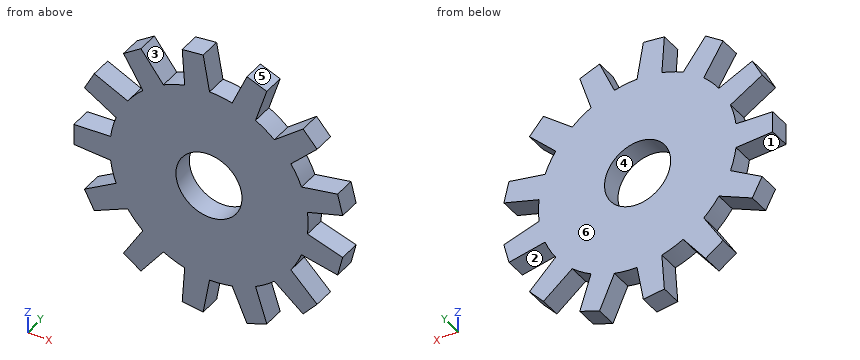
Autodesk Inventor part; units mm, degrees
ref_plane "YZ Plane" through (0, 0, 0) normal (1, 0, 0) x (0, 1, 0)
ref_plane "XZ Plane" through (0, 0, 0) normal (0, 1, 0) x (-1, 0, 0)
ref_plane "XY Plane" through (0, 0, 0) normal (0, 0, 1) x (1, 0, 0)
sketch "Szkic2" plane through (0, 0, 0) normal (0, 1, 0) x (-1, 0, 0)
  circle A0 centre (0, 0) radius 2.5
  circle A1 centre (0, 0) radius 10.25
  line L0 (10.2187, -0.8002) -> (10.2187, 0.8002)
  line L1 (10.2187, -0.8002) -> (7.4401, -0.9459)
  line L2 (10.2187, -0.8002) -> (13.0011, -0.8002) construction
  line L3 (10.2187, 0.8002) -> (7.4401, 0.9459)
  line L4 (10.2187, 0.8002) -> (13.0011, 0.8002) construction
  line L5 (9.4201, 4.0403) -> (7.0275, 2.6201)
  line L6 (8.6763, 5.4575) -> (6.1483, 4.2951)
  line L7 (9.4201, 4.0403) -> (8.6763, 5.4575)
  line L8 (6.4635, 7.9552) -> (5.0049, 5.5858)
  line L9 (5.1463, 8.8644) -> (3.448, 6.6604)
  line L10 (6.4635, 7.9552) -> (5.1463, 8.8644)
  line L11 (2.0261, 10.0477) -> (1.8358, 7.2719)
  line L12 (0.4373, 10.2407) -> (-0.0422, 7.4999)
  line L13 (2.0261, 10.0477) -> (0.4373, 10.2407)
  line L14 (-2.8754, 9.8384) -> (-1.7539, 7.292)
  line L15 (-4.3718, 9.2709) -> (-3.5227, 6.6212)
  line L16 (-2.8754, 9.8384) -> (-4.3718, 9.2709)
  line L17 (-7.1182, 7.3753) -> (-4.9418, 5.6417)
  line L18 (-8.1795, 6.1773) -> (-6.1962, 4.2257)
  line L19 (-7.1182, 7.3753) -> (-8.1795, 6.1773)
  line L20 (-9.7303, 3.2225) -> (-6.9976, 2.6989)
  line L21 (-10.1133, 1.6685) -> (-7.4503, 0.8622)
  line L22 (-9.7303, 3.2225) -> (-10.1133, 1.6685)
  line L23 (-10.1133, -1.6685) -> (-7.4503, -0.8622)
  line L24 (-9.7303, -3.2225) -> (-6.9976, -2.6989)
  line L25 (-10.1133, -1.6685) -> (-9.7303, -3.2225)
  line L26 (-8.1795, -6.1773) -> (-6.1962, -4.2257)
  line L27 (-7.1182, -7.3753) -> (-4.9418, -5.6417)
  line L28 (-8.1795, -6.1773) -> (-7.1182, -7.3753)
  line L29 (-4.3718, -9.2709) -> (-3.5227, -6.6212)
  line L30 (-2.8754, -9.8384) -> (-1.7539, -7.292)
  line L31 (-4.3718, -9.2709) -> (-2.8754, -9.8384)
  line L32 (0.4373, -10.2407) -> (-0.0422, -7.4999)
  line L33 (2.0261, -10.0477) -> (1.8358, -7.2719)
  line L34 (0.4373, -10.2407) -> (2.0261, -10.0477)
  line L35 (5.1463, -8.8644) -> (3.448, -6.6604)
  line L36 (6.4635, -7.9552) -> (5.0049, -5.5858)
  line L37 (5.1463, -8.8644) -> (6.4635, -7.9552)
  line L38 (8.6763, -5.4575) -> (6.1483, -4.2951)
  line L39 (9.4201, -4.0403) -> (7.0275, -2.6201)
  line L40 (8.6763, -5.4575) -> (9.4201, -4.0403)
  arc A2 (7.0275, -2.6201) -> (7.4401, -0.9459) centre (0, 0) ccw
  arc A3 (5.0049, -5.5858) -> (6.1483, -4.2951) centre (0, 0) ccw
  arc A4 (7.4401, 0.9459) -> (7.0275, 2.6201) centre (0, 0) ccw
  arc A5 (6.1483, 4.2951) -> (5.0049, 5.5858) centre (0, 0) ccw
  arc A6 (3.448, 6.6604) -> (1.8358, 7.2719) centre (0, 0) ccw
  arc A7 (-0.0422, 7.4999) -> (-1.7539, 7.292) centre (0, 0) ccw
  arc A8 (-3.5227, 6.6212) -> (-4.9418, 5.6417) centre (0, 0) ccw
  arc A9 (-6.1962, 4.2257) -> (-6.9976, 2.6989) centre (0, 0) ccw
  arc A10 (-7.4503, 0.8622) -> (-7.4503, -0.8622) centre (0, 0) ccw
  arc A11 (-6.9976, -2.6989) -> (-6.1962, -4.2257) centre (0, 0) ccw
  arc A12 (-4.9418, -5.6417) -> (-3.5227, -6.6212) centre (0, 0) ccw
  arc A13 (-1.7539, -7.292) -> (-0.0422, -7.4999) centre (0, 0) ccw
  arc A14 (1.8358, -7.2719) -> (3.448, -6.6604) centre (0, 0) ccw
  dimension "d58" = 5
  dimension "d60" = 20.5
  dimension "d61" = 177
  dimension "d62" = 177
  dimension "d65" = 360
extrude "Wyciągnięcie proste6" add sketch "Szkic2" along normal blind 1.6 contours L0 L1 A2 L39 L40 L38 A3 L36 L37 L35 A14 L33 L34 L32 A13 L30 L31 L29 A12 L27 L28 L26 A11 L24 L25 L23 A10 L21 L22 L20 A9 L18 L19 L17 A8 L15 L16 L14 A7 L12 L13 L11 A6 L9 L10 L8 A5 L6 L7 L5 A4 L3
properties part number "efektor zebatka1"
Geometry: final body of the model. Coordinates: model frame, mm. Face numbers are marked on the shaded views. A direction names the side the tool comes from. Coordinates: 2 decimals unless noted, no trailing zeros. Order: outer loops, then holes, each group sorted by start corner. A loop starts at its lowest first (then second) coordinate and runs counter-clockwise, first axis right, second up. Notation, with made-up numbers: (31, 11.25) -> (43, 11.25) arc R20 ccw to (43, 25.25) -> close; hole circle Ø7 at (62, 89.5). An arc over 180 degrees is marked (long way). Write each question's results on one line, items separated by ' | '. Start each with the question number.
1) Cut plane C-C, the plane z = -8.25. Output: boundary loops of the cut face in (x, y), and give its area (3 significant figures).
2) Cut plane A-A, the plane z = 0. Output: boundary loops of the cut face in (x, y).
3) Cut plane D-D, the plane x = -4.75. Output: boundary loops of the cut face in (y, z), and give its area (3 significant figures).
4) Set-up query: the marked faces 1, 2 and 3. Return all of +Z, -Z, +X, -X, +Y, -Y with unobstructed straight access to the full face (end or side cutting, diameter ignored); none if empty.
5) Mould query, pull axis Z, two halves, no side actions, for the marked faces 4, 5 and 6. Classes: released by +Z, released by -Z, zero draft, split by the parting line, or undercut.
6) Cut plane B-B, the plane x = 0.75. Output: boundary loops of the cut face in (y, z).
7) Material intervals for line 1 along Z through (x, y) = (-7.75, 0.5); line 2 along X through (y, z) = (1.25, 8.5); line 3 along Z through (x, y) = (7.25, 1.2), sorted ascending.
Checks:
1) outline: (-6.04, 0) -> (-4.67, 0) -> (-4.67, 1.6) -> (-6.04, 1.6) -> close; (-1.9, 0) -> (-0.09, 0) -> (-0.09, 1.6) -> (-1.9, 1.6) -> close; (2.18, 0) -> (4.04, 0) -> (4.04, 1.6) -> (2.18, 1.6) -> close | area: 8.07 mm^2
2) outline: (-10.22, 0) -> (-2.5, 0) -> (-2.5, 1.6) -> (-10.22, 1.6) -> close; (2.5, 0) -> (7.5, 0) -> (7.5, 1.6) -> (2.5, 1.6) -> close
3) outline: (0, -8.35) -> (1.6, -8.35) -> (1.6, 8.35) -> (0, 8.35) -> close | area: 26.7 mm^2
4) face 1: -X, +Y, -Y | face 2: +Y, -Y | face 3: +Z, +Y, -Y
5) face 4: undercut | face 5: released by +Z | face 6: zero draft
6) outline: (0, -7.46) -> (1.6, -7.46) -> (1.6, -2.38) -> (0, -2.38) -> close; (0, 2.38) -> (1.6, 2.38) -> (1.6, 7.46) -> (0, 7.46) -> close
7) line 1: -5.03 to -3.05, -0.93 to 0.93, 3.05 to 5.03 | line 2: -5.67 to -4.87, -1.92 to -0.13, 2.29 to 4.12 | line 3: -7.23 to -5.26, -2.75 to 2.75, 5.26 to 7.23
